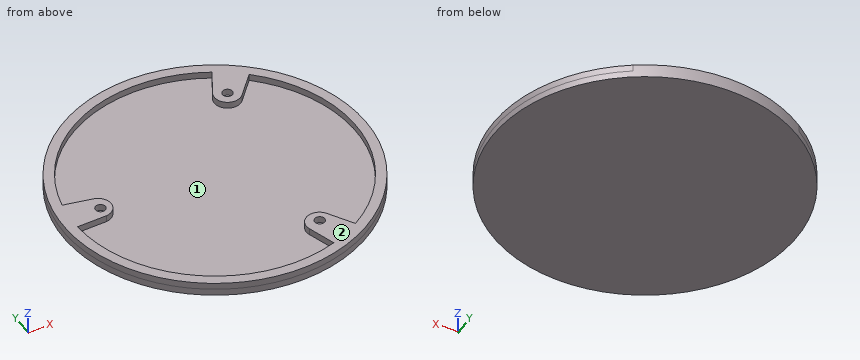
Autodesk Inventor part; units mm, degrees
ref_plane "YZ Plane" through (0, 0, 0) normal (1, 0, 0) x (0, 1, 0)
ref_plane "XZ Plane" through (0, 0, 0) normal (0, 1, 0) x (-1, 0, 0)
ref_plane "XY Plane" through (0, 0, 0) normal (0, 0, 1) x (1, 0, 0)
sketch "Esquisse1" plane through (0, 0, 0) normal (0, 0, 1) x (1, 0, 0)
  circle A0 centre (-32.9619, -13.3427) radius 1.5
  circle A1 centre (14.3997, -46.0802) radius 1.5
  circle A2 centre (19.4091, 11.459) radius 1.5
  arc A3 (-25, 21.4166) -> (25, 21.4166) centre (0, -16) ccw
  line L0 (25, 61) -> (25, 21.4166)
  line L1 (-25, 61) -> (25, 61)
  line L2 (-25, 21.4166) -> (-25, 61)
  circle A4 centre (0, -16) radius 42
  line L3 (0, -16) -> (24.2426, 18.2972) construction
  arc A5 (15.8278, 13.0403) -> (22.2865, 8.8044) centre (19.4091, 11.459) ccw
  line L4 (22.2865, 8.8044) -> (28.0705, 15.2418)
  line L5 (15.8278, 13.0403) -> (20.0997, 20.8782)
  line L6 (0, -16) -> (-41.8235, -12.1539) construction
  arc A6 (-33.0635, -16.8129) -> (-32.6245, -9.1015) centre (-33.4847, -12.9207) ccw
  line L7 (-32.6245, -9.1015) -> (-41.0914, -7.3112)
  line L8 (-33.0635, -16.8129) -> (-41.9873, -17.0323)
  line L9 (0, -16) -> (17.5809, -54.1433) construction
  arc A7 (17.2357, -44.2274) -> (10.338, -47.7029) centre (14.0756, -46.5383) ccw
  line L10 (10.338, -47.7029) -> (13.021, -55.9306)
  line L11 (17.2357, -44.2274) -> (21.8876, -51.8459)
  circle A8 centre (0, -16) radius 45
  point P0 (0, 0)
  point P1 (25, 21.4166)
  point P2 (-25, 21.4166)
  dimension "d0" = 3
  dimension "d3" = 360
extrude "Extrusion1" add sketch "Esquisse1" against normal blind 2 contours A8 A3 | L4 A5 L5 A4 | A4 L10 A7 L11 | L7 A6 L8 A4
sketch "Esquisse2" plane through (0, -16, -2) normal (0, 0, -1) x (-1, 0, 0)
  circle A0 centre (0, 0) radius 45
  point P0 (0, 16)
extrude "Extrusion2" add sketch "Esquisse2" along normal blind 2
properties part number "clips Anemo"
Source: CAD feature listing. Evaluate the final solid. Frame: model axes, mm. Face numbers are marked on the shaded views. Coordinates: 2 decimals unless noted, no trailing zeros. Write each loop counter-clockwise with the first axis right and the second up, starting at its lowest first coordinate (ties: lowest second). Pieces come first, ordered by that corner, then holes. Notation, with made-up numbers: (2, 40.5) -> (32, 40.5) arc R4 cw to (32, 46.5) -> close; hole circle Ø2 at (50.25, 54). An arc over 180 degrees is marked (long way). Return JSON: item names as keys, results as strings. Group by question number.
1) Ray query, line 1 along X through (y, z) = (-48.5, -1.8); line 2 along X through (y, z) = (-45, -1.5); line 3 along Z through (x, y) = (-23.5, -3). Return the intervals inside material, ascending.
2) Mould query, pull axis Y, two halves, no side actions, for the marked faces 1 and 2. Classes: +Y half, -Y half, draft (parallel to the pull), parting line (faces both ways), or undercut.
3) Section query A-A, the plane x = 0. Return loops of the section in (y, z).
4) Contact query for flat-ended pins moving along their axis: P1, Ø1.5, axis at y = -46, z = -3, coming from the +X side; P2, Ø1, axis at x = -20, y = 0.5, coming from the +Z side; P3, Ø1, axis at x = 14.5, z = -1, coming from the +Y side. Output: stop coordinate, or through.
5) Section query D-D, the plane x = -10.5. Return loops of the section in (y, z).
6) Section query C-C, the plane z = -2.8. Return loops of the section in (x, y), plus the area to 3 significant figures.
7) Section query B-B, the plane y = -29. Return loops of the section in (x, z).
From the geometry:
{
 "1": {"line 1": "-31.12 to -26.6, 10.6 to 19.84, 26.6 to 31.12", "line 2": "-34.41 to -30.38, 10.48 to 13.36, 15.44 to 17.71, 30.38 to 34.41", "line 3": "-4 to -2"},
 "2": {"face 1": "undercut", "face 2": "draft"},
 "3": {"outline": "(-61, -4) -> (29, -4) -> (29, 0) -> (26, 0) -> (26, -2) -> (-58, -2) -> (-58, 0) -> (-61, 0) -> close"},
 "4": {"P1": "x = 34.2", "P2": "z = -2", "P3": "y = 26.77"},
 "5": {"outline": "(-59.76, -4) -> (27.76, -4) -> (27.76, 0) -> (24.67, 0) -> (24.67, -2) -> (-56.67, -2) -> (-56.67, 0) -> (-59.76, 0) -> close"},
 "6": {"outline": "circle Ø90 at (0, -16)", "area": "6,360 mm²"},
 "7": {"outline": "(-43.08, -4) -> (43.08, -4) -> (43.08, 0) -> (39.94, 0) -> (39.94, -2) -> (-39.94, -2) -> (-39.94, 0) -> (-43.08, 0) -> close"}
}
